CAD build for the part. Positions are in the model's coordinates, mm. Face numbers are marked on the shaded views. A direction names the side the tool comes from. Round coordinates to 2 decimals unless told otherwise and drop trailing zeros. Loops run counter-clockwise (first coordinate to the right, second up) from the corner with the lowest first, then second, coordinate; pieces in that order, holes last. Notation, with made-up numbers: M -37,-29.5 L -9,-29.5 A10 ccw -9,-25.5 Z; hole C 10,21.5 d4. An arc over 180 degrees is marked long. Use one line per item in the form item = value.
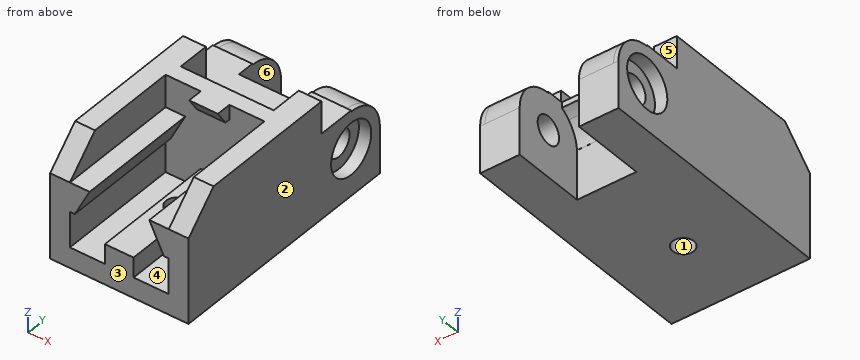
from build123d import *

# Parameters (mm, degrees)
SKETCH1_W                    = 26
SKETCH1_H                    = 28
BOSS_EXTRUDE1_DEPTH          = 50
CUT_EXTRUDE6_DEPTH           = 25
CUT_EXTRUDE3_DEPTH           = 39
SKETCH14_R                   = 7.5
BOSS_EXTRUDE7_DEPTH          = 7
SKETCH15_R                   = 2.8
CUT_EXTRUDE4_DEPTH           = 28
SKETCH16_R                   = 5.25
CUT_EXTRUDE5_DEPTH           = 1.5
CUT_EXTRUDE7_DEPTH           = 54.525694764
SKETCH19_R                   = 2.15
CUT_EXTRUDE9_DEPTH           = 50
ESQUISSE1_W                  = 12
ESQUISSE1_H                  = 9.5
ENL_V_MAT_EXTRU_1_DEPTH      = 7.5
ESQUISSE3_W                  = 12
ESQUISSE3_H                  = 7.5
ENL_V_MAT_EXTRU_3_DEPTH      = 10
BOSS_EXTRU_1_DEPTH           = 26
ENL_V_MAT_EXTRU_5_DEPTH      = 3.5
ESQUISSE9_W                  = 5.8
ESQUISSE9_H                  = 3
BOSS_EXTRU_3_DEPTH           = 1
BOSS_EXTRU_4_DEPTH           = 5.8
BOSS_EXTRU_5_DEPTH           = 0.1
BOSS_EXTRU_6_DEPTH           = 0.1
ESQUISSE13_W                 = 6.55
ESQUISSE13_H                 = 9.75
BOSS_EXTRU_7_DEPTH           = 3.6
ESQUISSE14_W                 = 6.55
ESQUISSE14_H                 = 9.75
BOSS_EXTRU_8_DEPTH           = 3.6
ESQUISSE16_R                 = 5.25
BOSS_EXTRU_9_DEPTH           = 1
BOSS_EXTRU_10_START          = 1
ESQUISSE17_R                 = 5.25
BOSS_EXTRU_10_DEPTH          = 1
ESQUISSE20_W                 = 4
ESQUISSE20_H                 = 25
BOSS_EXTRU_11_DEPTH          = 6.55
ENL_V_MAT_EXTRU_6_DEPTH      = 34
ENL_V_MAT_EXTRU_6_DEPTH_BACK = 10


with BuildPart() as part:
    # Sketch1 → Boss-Extrude1 (new body)
    with BuildSketch(Plane(origin=(0, 0, 0), x_dir=(1, 0, 0), z_dir=(0, 1, 0))):
        Rectangle(SKETCH1_W, SKETCH1_H)
    extrude(amount=BOSS_EXTRUDE1_DEPTH)

    # Sketch3 → Cut-Extrude6 (cut)
    with BuildSketch(Plane(origin=(0, 0, 0), x_dir=(1, 0, 0), z_dir=(0, 1, 0))):
        Polygon((9.998973293, 2.65), (9.998973293, 9.85), (2.900254006, 9.85), (2.881158298, 5.822816277), (-2.918777792, 5.850044076), (-2.9, 9.85), (-10, 9.85), (-10, 2.65), (-9, 2.65), (-6, -3.25), (-10, -3.25), (-10, -4.35), (-10, -15.089504782), (10.190019105, -15.10204882), (10.123266065, -8.899331206), (10.068921607, -3.849623622), (10.062468516, -3.25), (6.072889948, -3.25), (8.998973293, 2.65), align=None)
    extrude(amount=CUT_EXTRUDE6_DEPTH, mode=Mode.SUBTRACT)

    # Sketch7 → Cut-Extrude3 (cut)
    with BuildSketch(Plane(origin=(13, 0, 0), x_dir=(0, 0, -1), z_dir=(1, 0, 0))):
        with BuildLine():
            Line((4.5, 50), (-14, 50))
            Line((-14, 50), (-14, 24))
            Line((-14, 24), (-0.803300859, 37.196699141))
            ThreePointArc((-0.803300859, 37.196699141), (11.429096494, 39.629874257), (4.5, 50))
        make_face()
    extrude(amount=-CUT_EXTRUDE3_DEPTH, mode=Mode.SUBTRACT)

    # Sketch14 → Boss-Extrude7 (add)
    with BuildSketch(Plane(origin=(13, 0, 0), x_dir=(0, 0, -1), z_dir=(1, 0, 0))):
        with Locations((4.5, 42.5)):
            Circle(SKETCH14_R)
    boss_extrude7 = extrude(amount=-BOSS_EXTRUDE7_DEPTH)

    # Symétrie1: Boss-Extrude7 across plane
    add(boss_extrude7.mirror(Plane(origin=(0, 0, 0), x_dir=(0, 0, 1), z_dir=(1, 0, 0))))

    # Sketch15 → Cut-Extrude4 (cut)
    with BuildSketch(Plane(origin=(13, 0, 0), x_dir=(0, 0, -1), z_dir=(1, 0, 0))):
        with Locations((4.5, 42.5)):
            Circle(SKETCH15_R)
    extrude(amount=-CUT_EXTRUDE4_DEPTH, mode=Mode.SUBTRACT)

    # Sketch16 → Cut-Extrude5 (cut)
    with BuildSketch(Plane(origin=(13, 0, 0), x_dir=(0, 0, -1), z_dir=(1, 0, 0))):
        with Locations((4.5, 42.5)):
            Circle(SKETCH16_R)
    cut_extrude5 = extrude(amount=-CUT_EXTRUDE5_DEPTH, mode=Mode.SUBTRACT)

    # Mirror3: Cut-Extrude5 across plane
    add(cut_extrude5.mirror(Plane(origin=(0, 0, 0), x_dir=(0, 0, 1), z_dir=(1, 0, 0))), mode=Mode.SUBTRACT)

    # Sketch17 → Cut-Extrude7 (cut, through all)
    with BuildSketch(Plane.XZ):
        Polygon((-9.3, 3.25), (-13, 3.25), (-13, 14), (13, 14), (13, 3.25), (9.3, 3.25), (9.3, 9.8), (-9.3, 9.8), align=None)
    extrude(amount=-CUT_EXTRUDE7_DEPTH, mode=Mode.SUBTRACT)

    # Sketch19 → Cut-Extrude9 (cut)
    with BuildSketch(Plane(origin=(0, 0, -14), x_dir=(-1, 0, 0), z_dir=(0, 0, -1))):
        with Locations((0, 15)):
            Circle(SKETCH19_R)
    extrude(amount=-CUT_EXTRUDE9_DEPTH, mode=Mode.SUBTRACT)

    # Esquisse1 → Enlèv. mat.-Extru.1 (cut)
    with BuildSketch(Plane(origin=(0, 50, 0), x_dir=(1, 0, 0), z_dir=(0, 1, 0))):
        with Locations((0, 9.25)):
            Rectangle(ESQUISSE1_W, ESQUISSE1_H)
    extrude(amount=-ENL_V_MAT_EXTRU_1_DEPTH, mode=Mode.SUBTRACT)

    # Esquisse3 → Enlèv. mat.-Extru.3 (cut)
    with BuildSketch(Plane(origin=(0, 0, -14), x_dir=(-1, 0, 0), z_dir=(0, 0, -1))):
        with Locations((0, 38.75)):
            Rectangle(ESQUISSE3_W, ESQUISSE3_H)
    extrude(amount=-ENL_V_MAT_EXTRU_3_DEPTH, mode=Mode.SUBTRACT)

    # Esquisse6 → Boss.-Extru.1 (add)
    with BuildSketch(Plane(origin=(13, 0, 0), x_dir=(0, 0, -1), z_dir=(1, 0, 0))):
        with BuildLine():
            Line((-3.25, 34.75), (-3.25, 42.5))
            Line((-3.25, 42.5), (-3, 42.5))
            ThreePointArc((-3, 42.5), (-2.429096494, 39.629874257), (-0.803300859, 37.196699141))
            Line((-0.803300859, 37.196699141), (-3.25, 34.75))
        make_face()
    extrude(amount=-BOSS_EXTRU_1_DEPTH)

    # Esquisse7 → Enlèv. mat.-Extru.5 (cut)
    with BuildSketch(Plane(origin=(0, 42.5, 0), x_dir=(1, 0, 0), z_dir=(0, 1, 0))):
        Polygon((6, 3.615864876), (6, -7.096354864), (-6, -3.780069791), (-6, 8.456914553), align=None)
    extrude(amount=-ENL_V_MAT_EXTRU_5_DEPTH, mode=Mode.SUBTRACT)

    # Esquisse9 → Boss.-Extru.3 (add)
    with BuildSketch(Plane(origin=(0, 25, 0), x_dir=(-1, 0, 0), z_dir=(0, -1, 0))):
        with Locations((0, -8.3)):
            Rectangle(ESQUISSE9_W, ESQUISSE9_H)
    extrude(amount=BOSS_EXTRU_3_DEPTH)

    # Esquisse10 → Boss.-Extru.4 (add)
    with BuildSketch(Plane.ZY.offset(2.9)):
        Polygon((9.8, 24), (9.8, 22), (6.8, 24), align=None)
    extrude(amount=-BOSS_EXTRU_4_DEPTH)

    # Esquisse11 → Boss.-Extru.5 (add)
    with BuildSketch(Plane.ZY.offset(9.3)):
        Polygon((3.25, 34.75), (9.8, 28.2), (9.8, 25), (3.25, 25), align=None)
    extrude(amount=BOSS_EXTRU_5_DEPTH)

    # Esquisse12 → Boss.-Extru.6 (add)
    with BuildSketch(Plane(origin=(9.3, 0, 0), x_dir=(0, 0, -1), z_dir=(1, 0, 0))):
        Polygon((-9.8, 25), (-9.8, 28.2), (-3.25, 34.75), (-3.25, 25), align=None)
    extrude(amount=BOSS_EXTRU_6_DEPTH)

    # Esquisse13 → Boss.-Extru.7 (add)
    with BuildSketch(Plane(origin=(9.4, 0, 0), x_dir=(0, 0, -1), z_dir=(1, 0, 0))):
        with Locations((-6.525, 29.875)):
            Rectangle(ESQUISSE13_W, ESQUISSE13_H)
    extrude(amount=BOSS_EXTRU_7_DEPTH)

    # Esquisse14 → Boss.-Extru.8 (add)
    with BuildSketch(Plane.ZY.offset(9.4)):
        with Locations((6.525, 29.875)):
            Rectangle(ESQUISSE14_W, ESQUISSE14_H)
    extrude(amount=BOSS_EXTRU_8_DEPTH)

    # Esquisse16 → Boss.-Extru.9 (add)
    with BuildSketch(Plane.ZY.offset(13)):
        with BuildLine():
            Line((3.25, 0), (-14, 0))
            Line((-14, 0), (-14, 50))
            Line((-14, 50), (-4.5, 50))
            ThreePointArc((-4.5, 50), (0.803300859, 47.803300859), (3, 42.5))
            Line((3, 42.5), (3.25, 42.5))
            Line((3.25, 42.5), (3.25, 34.75))
            Line((3.25, 34.75), (9.8, 34.75))
            Line((9.8, 34.75), (9.8, 25))
            Line((9.8, 25), (3.25, 25))
            Line((3.25, 25), (3.25, 0))
        make_face()
        with Locations(Location((-4.5, 42.5, 0), (0, 0, 180))):
            Circle(ESQUISSE16_R, mode=Mode.SUBTRACT)
    extrude(amount=BOSS_EXTRU_9_DEPTH)

    # Esquisse17 → Boss.-Extru.10 (add)
    with BuildSketch(Plane(origin=(13, 0, 0), x_dir=(0, 0, -1), z_dir=(1, 0, 0)).offset(BOSS_EXTRU_10_START)):
        with BuildLine():
            Line((-3, 42.5), (-3.25, 42.5))
            Line((-3.25, 42.5), (-3.25, 34.75))
            Line((-3.25, 34.75), (-9.8, 34.75))
            Line((-9.8, 34.75), (-9.8, 25))
            Line((-9.8, 25), (-3.25, 25))
            Line((-3.25, 25), (-3.25, 0))
            Line((-3.25, 0), (14, 0))
            Line((14, 0), (14, 50))
            Line((14, 50), (4.5, 50))
            ThreePointArc((4.5, 50), (-0.803300859, 47.803300859), (-3, 42.5))
        make_face()
        with Locations((4.5, 42.5)):
            Circle(ESQUISSE17_R, mode=Mode.SUBTRACT)
    extrude(amount=-BOSS_EXTRU_10_DEPTH)

    # Esquisse20 → Boss.-Extru.11 (add)
    with BuildSketch(Plane.XY.offset(3.25)):
        with Locations((-12, 12.5)):
            Rectangle(ESQUISSE20_W, ESQUISSE20_H)
        with Locations((12, 12.5)):
            Rectangle(ESQUISSE20_W, ESQUISSE20_H)
    extrude(amount=BOSS_EXTRU_11_DEPTH)

    # Esquisse22 → Enlèv. mat.-Extru.6 (cut, two sides: drawn at the far end of the back side and taken through both)
    with BuildSketch(Plane.ZY.offset(-10).offset(-ENL_V_MAT_EXTRU_6_DEPTH_BACK)):
        Polygon((3.25, 0), (9.8, 6.55), (13.122553289, -3.826398857), (3.25, -3.616824535), align=None)
    extrude(amount=ENL_V_MAT_EXTRU_6_DEPTH + ENL_V_MAT_EXTRU_6_DEPTH_BACK, mode=Mode.SUBTRACT)


solid = part.part
1. Pull direction Y, two halves, no side cores. Call the marked faces 1, 2 and 3: +Y half, -Y half, draft (parallel to the pull), parting line (faces both ways), or undercut.
Completed:
face_1 = undercut
face_2 = draft
face_3 = -Y half
2. Cut at D-D on z = 6.25. Write the cut outline in (x, y), and give its area (3 significant figures).
Completed:
outline = M -14,3 L -10,3 L -10,25 L 10,25 L 10,3 L 14,3 L 14,34.75 L 9.4,34.75 L 9.4,31.75 L -9.4,31.75 L -9.4,34.75 L -14,34.75 Z
area = 393 mm2
3. Cut at A-A on z = -12.25. Write the cut outline in (x, y).
Completed:
outline = M -14,0 L 14,0 L 14,50 L 6,50 L 6,35 L -6,35 L -6,50 L -14,50 Z; hole C 0,15 d4.3
4. Probe line 1 along X through (y, z) = (36.5, -5.5); line 2 along Y through (x, z) = (9.2, -4.5); line 3 along Y through (x, z) = (0, -8.5). List the from-to ranges inside material, lowest first. Write a range as from..to.
Completed:
line_1 = -14..-6, 6..14
line_2 = 25..39.7, 45.3..50
line_3 = 0..12.85, 17.15..35
5. Cut at B-B on x = 12.25. Write the cut outline in (y, z).
Completed:
outline = M 0,-14 L 50,-14 L 50,-4.5 A7.5 ccw 42.5,3 L 42.5,3.25 L 34.75,3.25 L 34.75,9.8 L 6.55,9.8 L 0,3.25 Z; hole C 42.5,-4.5 d10.5
6. Drop flat-ended pins along their axis: P1, Ø5, axis at x = 8, z = -9, coming from the -Y side; P2, Ø1.2, axis at x = -7, y = 17, coming from the +Z side; P3, Ø7.5, axis at y = 42.5, z = -4.5, coming from the -X side; P4, Ø5, axis at y = 44.5, z = -4, coming from the +X side. Give the stop position or say it passes through.
Completed:
P1 = 0
P2 = 3.25
P3 = -11.5
P4 = 11.5
7. Tool access for the marked faces 4, 5 and 6: list every direction of +Z, -Z, +X, -X, +Y, -Y with a clear straight run to the whole face (end or side of a thin tool).
Completed:
face_4 = -Y
face_5 = +Z, +X, -X, +Y
face_6 = -Z, +Y
8. Cut at C-C on y = 15. Write the cut outline in (x, z).
Completed:
outline = M -14,-14 L -2.15,-14 L -2.15,-5.85 L -2.92,-5.85 L -2.9,-9.85 L -10,-9.85 L -10,-2.65 L -9,-2.65 L -6,3.25 L -10,3.25 L -10,9.8 L -14,9.8 Z; M 2.15,-14 L 14,-14 L 14,9.8 L 10,9.8 L 10,3.25 L 6.07,3.25 L 9,-2.65 L 10,-2.65 L 10,-9.85 L 2.9,-9.85 L 2.88,-5.82 L 2.15,-5.83 Z
